Autodesk Inventor part; units mm, degrees
ref_plane "YZ Plane" through (0, 0, 0) normal (1, 0, 0) x (0, 1, 0)
ref_plane "XZ Plane" through (0, 0, 0) normal (0, 1, 0) x (-1, 0, 0)
ref_plane "XY Plane" through (0, 0, 0) normal (0, 0, 1) x (1, 0, 0)
sketch "Sketch1" plane through (0, 0, 0) normal (0, 0, 1) x (1, 0, 0)
  line L0 (12.7, -25.4) -> (-12.7, -25.4)
  line L1 (-12.7, -25.4) -> (-12.7, 25.4)
  line L2 (-12.7, 25.4) -> (12.7, 25.4)
  line L3 (12.7, 25.4) -> (12.7, -25.4)
  line L4 (12.7, -25.4) -> (-12.7, 25.4) construction
  line L5 (-12.7, -25.4) -> (12.7, 25.4) construction
  line L6 (10.16, 22.86) -> (-10.16, 22.86)
  line L7 (-10.16, 22.86) -> (-10.16, -22.86)
  line L8 (-10.16, -22.86) -> (10.16, -22.86)
  line L9 (10.16, -22.86) -> (10.16, 22.86)
  point P0 (0, 0)
  dimension "d0" = 25.4
  dimension "d1" = 50.8
  dimension "d2" = 2.54
extrude "Extrusion1" add sketch "Sketch1" along normal mid plane 355.6
sketch "Sketch2" plane through (-12.7, 25.4, 177.8) normal (0, 1, 0) x (1, 0, 0)
  point P0 (12.7, 177.8)
  point P1 (12.7, 190.5)
  point P2 (12.7, 165.1)
  dimension "HoleOffset" = 12.7
  dimension "d6" = 12.7
hole "Hole1" at (0, 25.4, -12.7) at (0, 25.4, 12.7) direction (0, -1, 0) diameter 4.1656 end through all
pattern_linear "Rectangular Pattern1" count 31 spacing 50.8 along (0, 0, 1) of "Hole1" first direction both ways yes
properties part number "VersaFrame Side Rail" material "Aluminum 6061"
Check sheet for the modelled part. Datum: model origin and axes. Units: mm. A direction names the side the tool comes from. Coordinates: 2 decimals unless noted, no trailing zeros. Write each loop counter-clockwise with the first axis right and the second up, starting at its lowest first coordinate (ties: lowest second). Pieces come first, ordered by that corner, then holes.
Item 1: Depth check by flat-ended pin: pin 1 Ø6 at (x, y) = (-10, 16.5) entering from +Z. Enter the tip coordinate at first touch or a pass-through.
Numbers:
pin 1: stops at z = 177.8
Item 2: Cross-section at A-A on y = 16.5. Record the boundary of the cut face in (x, z).
Numbers:
outline: (-12.7, -177.8) - (-10.16, -177.8) - (-10.16, 177.8) - (-12.7, 177.8) - close; (10.16, -177.8) - (12.7, -177.8) - (12.7, 177.8) - (10.16, 177.8) - close
Item 3: Mould release check, pull along X, two halves, no side actions. Record for faces 1 (the face through (12.7, 0, -2)), 2 (the face through (-10.4, 2, 177.8)), 3 (the face through (-10.16, 0, -2)): released by +X, released by -X, zero draft, split by the parting line, or undercut.
Numbers:
face 1: released by +X
face 2: zero draft
face 3: undercut
Item 4: Scan lines: probe 1 along Y at (x, z) = (-2, -50); probe 2 along X at (y, z) = (-17.5, -91); probe 3 along X at (y, z) = (-24, -38). Record each from-to range of solid material in increasing order.
Numbers:
probe 1: y = -25.4 to -22.86, 22.86 to 25.4
probe 2: x = -12.7 to -10.16, 10.16 to 12.7
probe 3: x = -12.7 to -2.08, 2.08 to 12.7
Item 5: Access from +Z, -Z, +X, -X, +Y, -Y to the whole of each face (thin tool, end or side, straight path). Record for faces 4 (the face through (0, -22.86, -2)), 5 (the face through (0, -25.4, -2)).
Numbers:
face 4: +Z, -Z
face 5: +Z, -Z, +X, -X, -Y
Item 6: Cross-section at B-B on z = 54.5. Record the boundary of the cut face in (x, y).
Numbers:
outline: (-12.7, -25.4) - (12.7, -25.4) - (12.7, 25.4) - (-12.7, 25.4) - close; hole (-10.16, -22.86) - (10.16, -22.86) - (10.16, 22.86) - (-10.16, 22.86) - close
